Read the model definition and answer for the solid it produces. Units are mm, in the model's axes. A direction names the side the tool comes from. Give positions to 0.01 mm unless a question says otherwise; leave off trailing zeros. Order: outer loops, then holes, each group sorted by start corner. A loop starts at its lowest first (then second) coordinate and runs counter-clockwise, first axis right, second up. Notation, with made-up numbers: (-11, 88.5) - (9, 88.5) arc R26 cw to (9, 105.5) - close; hole circle Ø7 at (5, -3). An arc over 180 degrees is marked (long way). Return JSON: item names as keys, results as strings.
```python
from build123d import *

# Parameters (mm, degrees)
F0_W = 10
F0_H = 0.5


with BuildPart() as f1:
    # F0 (on Front) → F1 (revolve)
    with BuildSketch(Plane.XZ):
        Polygon((0, 11.912), (-32.248389, 11.912), (-32.248389, 11.412), (-32.248389, 10.912), (0, 10.912), align=None)
        Polygon((37.701611, 11.912), (0, 11.912), (0, 10.912), (37.701611, 10.912), (37.701611, 11.412), align=None)
        with Locations((-37.248389, 11.162)):
            Rectangle(F0_W, F0_H)
        with Locations((42.701611, 11.662)):
            Rectangle(F0_W, F0_H)
    revolve(axis=Axis((18.951043, 0, 0), (1, 0, 0)))


solid = f1.part
```
Q1. A cutting plane is placed at A-A (z = 0). Write down the section's boundary in (x, y), and give its area (3 significant figures).
Values:
{"outline": "(-42.25, -11.41) - (-32.25, -11.41) - (-32.25, -11.91) - (47.7, -11.91) - (47.7, -11.41) - (37.7, -11.41) - (37.7, -10.91) - (-42.25, -10.91) - close; (-42.25, 10.91) - (37.7, 10.91) - (37.7, 11.41) - (47.7, 11.41) - (47.7, 11.91) - (-32.25, 11.91) - (-32.25, 11.41) - (-42.25, 11.41) - close", "area": "160 mm²"}
Q2. Consider L1, parallel to Z at x = 40.5, y = 0; L2, parallel to Y at x = 2, z = 0. Determine where each line is inside the solid, lowest interval first.
Values:
{"L1": "z = -11.91 to -11.41, 11.41 to 11.91", "L2": "y = -11.91 to -10.91, 10.91 to 11.91"}
Q3. Determine the mould class of faces 3 (the cylindrical face through (42.77, 6.94, -9.06)), 4 (the cylindrical face through (7.17, -3.58, 11.36)), 5 (the flat face through (47.702, 6, -10)) for opening direction Z: released by +Z, released by -Z, zero draft, split by the parting line, or undercut.
Values:
{"face 3": "undercut", "face 4": "split by the parting line", "face 5": "zero draft"}
Q4. Given pin 1 (4 mm diameter, centred on x = -30, y = 9, fed in from -Z); pin 2 (1.5 mm diameter, centred on x = 12.5, z = -9.5, fed in from +Y); pin 3 (10 mm diameter, centred on x = -11, z = -5.5, fed in from -Y); pin 4 (12 mm diameter, centred on y = 2.5, z = -2, fed in from -X), each flat-ended and moving along its own axis, determine where each tip first touches the part or whether it passes through.
Values:
{"pin 1": "stops at z = -9.64", "pin 2": "stops at y = 8.08", "pin 3": "stops at y = -11.9", "pin 4": "passes through"}
Q5. For faces 1 (the cylindrical face through (-1.7, -3.3, 10.4)), 2 (the flat face through (-32.248, 6, 10)), determine the directions among +Z, -Z, +X, -X, +Y, -Y from which every point of the face is accessible in a straight line to the end or side of a thin tool.
Values:
{"face 1": "+X, -X", "face 2": "-X"}
Q6. A cutting plane is placed at D-D (x = 19.5). Write down the section's boundary in (y, z).
Values:
{"outline": "circle Ø23.82 at (0, 0); hole circle Ø21.82 at (0, 0)"}
Q7. A cutting plane is placed at C-C (x = 39). Write down the section's boundary in (y, z).
Values:
{"outline": "circle Ø23.82 at (0, 0); hole circle Ø22.82 at (0, 0)"}
